Check sheet for the modelled part. Datum: model origin and axes. Units: mm. Face numbers are marked on the shaded views. A direction names the side the tool comes from. Round coordinates to 2 decimals unless told otherwise and drop trailing zeros. Loops run counter-clockwise (first coordinate to the right, second up) from the corner with the lowest first, then second, coordinate; pieces in that order, holes last. Notation, with made-up numbers: (-0.75, 81) -> (9.25, 81) arc R29 cw to (9.25, 110) -> close; hole circle Ø7 at (3.5, 85.5). An arc over 180 degrees is marked (long way). Return JSON: item names as keys, results as strings.
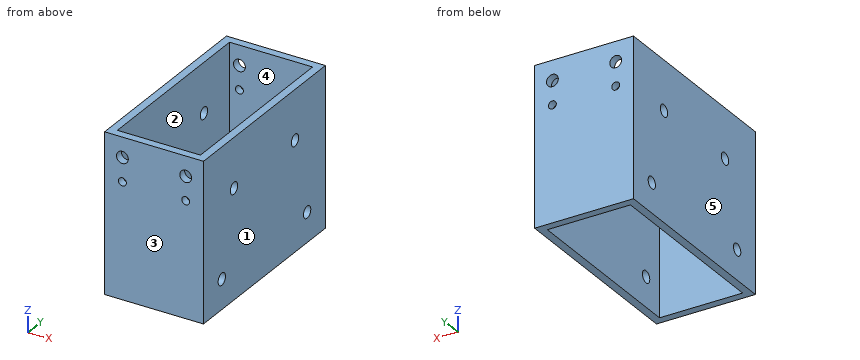
Autodesk Inventor part; units mm, degrees
ref_plane "YZ Plane" through (0, 0, 0) normal (1, 0, 0) x (0, 1, 0)
ref_plane "XZ Plane" through (0, 0, 0) normal (0, 1, 0) x (-1, 0, 0)
ref_plane "XY Plane" through (0, 0, 0) normal (0, 0, 1) x (1, 0, 0)
sketch "スケッチ1" plane through (0, 0, 0) normal (0, 0, 1) x (1, 0, 0)
  line L0 (-12.5, 25) -> (12.5, 25)
  line L1 (12.5, 25) -> (12.5, -25)
  line L2 (12.5, -25) -> (-12.5, -25)
  line L3 (-12.5, -25) -> (-12.5, 25)
  line L4 (-10.5, 23) -> (10.5, 23)
  line L5 (10.5, 23) -> (10.5, -23)
  line L6 (10.5, -23) -> (-10.5, -23)
  line L7 (-10.5, -23) -> (-10.5, 23)
  point P0 (0, 0)
  dimension "d0" = 21
  dimension "d2" = 25
  dimension "d3" = 10.5
  dimension "d4" = 46
  dimension "d5" = 50
  dimension "d6" = 23
  dimension "d7" = 25
  dimension "d8" = 12.5
extrude "押し出し1" add sketch "スケッチ1" against normal blind 40
sketch "スケッチ2" plane through (-12.5, 25, 0) normal (0, 1, 0) x (1, 0, 0)
  line L0 (0, 0) -> (25, 0)
  line L1 (0, 0) -> (0, 40)
  circle A0 centre (4.5, 5) radius 1.5
  circle A1 centre (20.5, 5) radius 1.5
  point P0 (12.5, 0)
  dimension "d13" = 3
  dimension "d14" = 16
  dimension "d16" = 4.5
  dimension "d18" = 5
  dimension "d21" = 5
hole "穴1" at (8, 25, -5) at (-8, 25, -5) direction (0, -1, 0) diameter 3 end through all
sketch "スケッチ3" plane through (-12.5, 25, 0) normal (0, 1, 0) x (1, 0, 0)
  circle A0 centre (20.5, 5) radius 1.5
  circle A1 centre (4.5, 5) radius 1.5
  line L0 (0, 0) -> (0, 40)
  circle A2 centre (4.5, 11) radius 1
  circle A3 centre (20.5, 11) radius 1
  point P0 (12.5, 0)
  dimension "d29" = 2
  dimension "d31" = 16
  dimension "d32" = 4.5
  dimension "d33" = 6
  dimension "d34" = 6
hole "穴2" at (8, 25, -11) at (-8, 25, -11) direction (0, -1, 0) diameter 2 end through all
sketch "スケッチ4" plane through (12.5, -25, 0) normal (1, 0, 0) x (0, 0, -1)
  line L0 (0, 0) -> (40, 0)
  line L1 (40, 50) -> (40, 0)
  circle A0 centre (32.5, 42.5) radius 1.5
  circle A1 centre (32.5, 7.5) radius 1.5
  circle A2 centre (12.5, 12.5) radius 1.5
  circle A3 centre (12.5, 37.5) radius 1.5
  point P0 (0, 25)
  dimension "d42" = 3
  dimension "d44" = 25
  dimension "d45" = 35
  dimension "d46" = 7.5
  dimension "d47" = 12.5
  dimension "d48" = 20
  dimension "d49" = 20
  dimension "d50" = 7.5
  dimension "d51" = 7.5
hole "穴3" at (12.5, -12.5, -12.5) at (12.5, -17.5, -32.5) at (12.5, 17.5, -32.5) at (12.5, 12.5, -12.5) direction (-1, 0, 0) diameter 3 end through all
properties part number "Pitch_Free_Case"
Q1. Tool access check on the marked faces 1 and 2. Record the directions out of +Z, -Z, +X, -X, +Y, -Y that give a thin tool (end or side, any length) a straight path to the whole face; none if there is none.
Results list:
{"face 1": "+Z, -Z, +X, +Y, -Y", "face 2": "+Z, -Z"}
Q2. Material ranges on line 1 (X direction, y = 24.3, z = -5); line 2 (Z direction, x = 8, y = -24.1); line 3 (Y direction, x = 11.4, z = -32.5), recorded low to high.
Results list:
{"line 1": "-12.5 to -9.5, -6.5 to 6.5, 9.5 to 12.5", "line 2": "-40 to -12, -10 to -6.5, -3.5 to 0", "line 3": "-25 to -19, -16 to 16, 19 to 25"}
Q3. Section check C-C (z = -25). Record the boundary of the cut face in (x, y), then the cut area to 3 significant figures.
Results list:
{"outline": "(-12.5, -25) -> (12.5, -25) -> (12.5, 25) -> (-12.5, 25) -> close; hole (-10.5, -23) -> (10.5, -23) -> (10.5, 23) -> (-10.5, 23) -> close", "area": "284 mm^2"}
Q4. Section check B-B (x = -1.5). Record the boundary of the cut face in (y, z).
Results list:
{"outline": "(-25, -40) -> (-23, -40) -> (-23, 0) -> (-25, 0) -> close; (23, -40) -> (25, -40) -> (25, 0) -> (23, 0) -> close"}
Q5. Section check A-A (y = -12.5). Record the boundary of the cut face in (x, z).
Results list:
{"outline": "(-12.5, -40) -> (-10.5, -40) -> (-10.5, -14) -> (-12.5, -14) -> close; (-12.5, -11) -> (-10.5, -11) -> (-10.5, 0) -> (-12.5, 0) -> close; (10.5, -40) -> (12.5, -40) -> (12.5, -14) -> (10.5, -14) -> close; (10.5, -11) -> (12.5, -11) -> (12.5, 0) -> (10.5, 0) -> close"}
Q6. Go/stop test with a flat-tipped pin: pin 1 (1.8 mm diameter, centred on x = -8, z = -11, fed in from +Y). Record where the tip stops, or that it passes through.
Results list:
{"pin 1": "through"}
Q7. Section check D-D (z = -5). Record the boundary of the cut face in (x, y).
Results list:
{"outline": "(-12.5, -25) -> (-9.5, -25) -> (-9.5, -23) -> (-10.5, -23) -> (-10.5, 23) -> (-9.5, 23) -> (-9.5, 25) -> (-12.5, 25) -> close; (-6.5, -25) -> (6.5, -25) -> (6.5, -23) -> (-6.5, -23) -> close; (-6.5, 23) -> (6.5, 23) -> (6.5, 25) -> (-6.5, 25) -> close; (9.5, -25) -> (12.5, -25) -> (12.5, 25) -> (9.5, 25) -> (9.5, 23) -> (10.5, 23) -> (10.5, -23) -> (9.5, -23) -> close"}
Q8. Draft check along X on the marked faces 3, 4 and 5. Enter one of: released by +X, released by -X, zero draft, split by the parting line, or undercut.
Results list:
{"face 3": "zero draft", "face 4": "undercut", "face 5": "released by -X"}
